from build123d import *

# Parameters (mm, degrees)
SKETCH_1_R       = 2.9
EXTRUDE_1_DEPTH  = 4
CHAMFER_1_SIZE   = 0.6
SKETCH_3_W       = 12
SKETCH_3_H       = 19.86
EXTRUDE_2_DEPTH  = 2
SKETCH_4_W       = 10
SKETCH_4_H       = 12
SKETCH_4_R       = 1.6
EXTRUDE_3_DEPTH  = 3
FILLET_START     = -15
FILLET_2_DEPTH   = 4.14
FILLET_START_2   = -13.86
FILLET_2_2_DEPTH = 3
SKETCH_5_W       = 46
SKETCH_5_H       = 19.86
SKETCH_5_R       = 1.5
EXTRUDE_4_DEPTH  = 1
CHAMFER_4_SIZE   = 1


with BuildPart() as part:
    # 草图1 → 凸台-拉伸1 (new body)
    with BuildSketch(Plane.XY):
        Polygon((7.937253933, 6), (-21, 6), (-21, -13.86), (7.937253933, -13.86), (21, -13.86), (21, 6), align=None)
        Circle(SKETCH_1_R, mode=Mode.SUBTRACT)
    extrude(amount=EXTRUDE_1_DEPTH)

    # 倒角1
    chamfer_1_edges = [part.edges().sort_by_distance(p)[0] for p in [
        (-2.9, 0, 4),
    ]]
    chamfer(chamfer_1_edges, length=CHAMFER_1_SIZE)

    # 草图3 → 凸台-拉伸2 (add)
    with BuildSketch(Plane.ZY.offset(21)):
        with Locations((6, -3.93)):
            Rectangle(SKETCH_3_W, SKETCH_3_H)
    extrude_2 = extrude(amount=EXTRUDE_2_DEPTH)

    # 镜向1: 凸台-拉伸2 across plane
    add(extrude_2.mirror(Plane(origin=(0, 0, 0), x_dir=(0, 0, 1), z_dir=(1, 0, 0))))

    # 草图4 → 凸台-拉伸3 (add)
    # profile 1 of 2: a face of its own
    with BuildSketch(Plane.XZ.offset(13.86)):
        with Locations((-18, 6)):
            Rectangle(SKETCH_4_W, SKETCH_4_H)
        with Locations((-17, 8)):
            Circle(SKETCH_4_R, mode=Mode.SUBTRACT)
    # profile 2 of 2: a face of its own
    with BuildSketch(Plane.XZ.offset(13.86)):
        with Locations((18, 6)):
            Rectangle(SKETCH_4_W, SKETCH_4_H)
        with Locations(Location((17, 8, 0), (0, 0, 180))):
            Circle(SKETCH_4_R, mode=Mode.SUBTRACT)
    extrude(amount=-EXTRUDE_3_DEPTH)

    # 圆角2: read off the stored shape, not the designer's step
    # 圆角2 outline → 圆角2 (cut)
    with BuildSketch(Plane(origin=(0, 0, 0), x_dir=(1, 0, 0), z_dir=(0, 1, 0)).offset(FILLET_START)):
        with BuildLine():
            Line((13, -12), (17, -12))
            ThreePointArc((17, -12), (14.171572875, -10.828427125), (13, -8))
            Line((13, -8), (13, -12))
        make_face()
        with BuildLine():
            Line((-13, -12), (-13, -8))
            ThreePointArc((-13, -8), (-14.171572875, -10.828427125), (-17, -12))
            Line((-17, -12), (-13, -12))
        make_face()
    extrude(amount=FILLET_2_DEPTH, mode=Mode.SUBTRACT)

    # Fillet 2 2 outline → Fillet 2 2 (add)
    with BuildSketch(Plane(origin=(0, 0, 0), x_dir=(1, 0, 0), z_dir=(0, 1, 0)).offset(FILLET_START_2)):
        with BuildLine():
            ThreePointArc((-13, -8), (-11.828427125, -5.171572875), (-9, -4))
            Line((-9, -4), (-13, -4))
            Line((-13, -4), (-13, -8))
        make_face()
        with BuildLine():
            ThreePointArc((9, -4), (11.828427125, -5.171572875), (13, -8))
            Line((13, -8), (13, -4))
            Line((13, -4), (9, -4))
        make_face()
    extrude(amount=FILLET_2_2_DEPTH)

    # 草图5 → 凸台-拉伸4 (add)
    with BuildSketch(Plane(origin=(0, 0, 0), x_dir=(-1, 0, 0), z_dir=(0, 0, -1))):
        with Locations((0, -3.93)):
            Rectangle(SKETCH_5_W, SKETCH_5_H)
        Circle(SKETCH_5_R, mode=Mode.SUBTRACT)
    extrude(amount=EXTRUDE_4_DEPTH)

    # 倒角4
    chamfer_4_edges = [part.edges().sort_by_distance(p)[0] for p in [
        (0, 6, -1),
        (23, -3.93, -1),
        (0, -13.86, -1),
        (-23, 6, 5.5),
        (-23, -13.86, 5.5),
        (23, -13.86, 5.5),
        (23, 6, 5.5),
        (-21, -2.43, 4),
    ]]
    chamfer(chamfer_4_edges, length=CHAMFER_4_SIZE)


solid = part.part
Model file for the job. Use its own axes, mm. A direction names the side the tool comes from. Give positions to 0.01 mm unless a question says otherwise; leave off trailing zeros. Loops run counter-clockwise (first coordinate to the right, second up) from the corner with the lowest first, then second, coordinate; pieces in that order, holes last.
1) Flat gauge pins, fed straight in: pin 1 Ø3.5 at (x, y) = (0, 0) entering from +Z; pin 2 Ø2.5 at (x, z) = (17, 6.5) entering from +Y; pin 3 Ø1.8 at (x, y) = (0, 0) entering from -Z; pin 4 Ø1.5 at (x, y) = (2, -9) entering from +Z. Where does each tip first touch, or does it go through?
2) Tool access for faces 1 (the cylindrical face through (18.27, -12.38, 8.97)), 2 (the flat face through (-20.5, -2.3, 4.5)): list every direction of +Z, -Z, +X, -X, +Y, -Y with a clear straight run to the whole face (end or side of a thin tool).
3) Wall check: line 1 (X direction, y = 1.75, z = 6.25); line 2 (Z direction, x = -9, y = 1); line 3 (Y direction, x = -15, z = 5.25). Give the ranges that are in metal, low to high.
4) Saw through at B-B (y = -11.75). Write the cut outline in (x, z).
5) Saw through at D-D (x = 0). Write the cut outline in (y, z), plus the area to 3 significant figures.
6) Saw through at A-A (z = 1.75). Write the cut outline in (x, y).
7) Pull direction Y, two halves, no side cores. Call faces 3 (the flat face through (22.3, -13.24, -0.32)), 4 (the flat face through (-1.2, -1.2, 0)), 5 (the flat face through (-16, -10.86, 6)), 6 (the flat face through (-23, -4, 6)): +Y half, -Y half, draft (parallel to the pull), parting line (faces both ways), or undercut.
8) Saw through at C-C (y = 0). Write the cut outline in (x, z), plus the area to 3 significant figures.
Answer block:
1. pin 1: stops at z = 0
1. pin 2: stops at y = -10.86
1. pin 3: passes through
1. pin 4: stops at z = 4
2. face 1: +Y, -Y
2. face 2: +Z, +Y
3. line 1: x = -23 to -21, 21 to 23
3. line 2: z = -1 to 4
3. line 3: y = -13.86 to -10.86
4. outline: (-23, -1) - (22, -1) - (23, 0) - (23, 12) - (17, 12) arc R4 ccw to (13, 8) arc R4 cw to (9, 4) - (-9, 4) arc R4 cw to (-13, 8) arc R4 ccw to (-17, 12) - (-23, 12) - close; hole circle Ø3.2 at (-17, 8); hole circle Ø3.2 at (17, 8)
5. outline: (-13.86, 0) - (-12.86, -1) - (-1.5, -1) - (-1.5, 0) - (-2.9, 0) - (-2.9, 3.4) - (-3.5, 4) - (-13.86, 4) - close; (1.5, -1) - (5, -1) - (6, 0) - (6, 4) - (3.5, 4) - (2.9, 3.4) - (2.9, 0) - (1.5, 0) - close
5. area: 71.7 mm2
6. outline: (-23, -12.86) - (-22, -13.86) - (22, -13.86) - (23, -12.86) - (23, 5) - (22, 6) - (-22, 6) - (-23, 5) - close; hole circle Ø5.8 at (0, 0)
7. face 3: -Y half
7. face 4: undercut
7. face 5: +Y half
7. face 6: draft
8. outline: (-23, -1) - (-1.5, -1) - (-1.5, 0) - (-2.9, 0) - (-2.9, 3.4) - (-3.5, 4) - (-20, 4) - (-21, 5) - (-21, 12) - (-23, 12) - close; (1.5, -1) - (22, -1) - (23, 0) - (23, 12) - (21, 12) - (21, 4) - (3.5, 4) - (2.9, 3.4) - (2.9, 0) - (1.5, 0) - close
8. area: 235 mm2
